from build123d import *
from build123d.topology import SkipClean

# Parameters (mm, degrees)
SKETCH2_R           = 18.921523051
SKETCH2_R_2         = 3.4
BOSS_EXTRUDE1_DEPTH = 10
FILLET1_R           = 3
SKETCH3_R           = 18.921523051
SKETCH3_R_2         = 3.4
BOSS_EXTRUDE2_DEPTH = 0.5
SKETCH4_R           = 18.921523051
BOSS_EXTRUDE3_DEPTH = 5
SKETCH8_R           = 18.921523051
BOSS_EXTRUDE4_DEPTH = 15
SKETCH10_R          = 4.25
CUT_EXTRUDE2_DEPTH  = 40
FILLET2_R           = 10
SKETCH11_R          = 3.4
CUT_EXTRUDE3_DEPTH  = 10.5


with BuildPart() as part:
    # Sketch2 → Boss-Extrude1 (new body)
    with BuildSketch(Plane.XY):
        Circle(SKETCH2_R)
        with Locations((0, 11.25277675)):
            Circle(SKETCH2_R_2, mode=Mode.SUBTRACT)
        with Locations((11.25277675, 0)):
            Circle(SKETCH2_R_2, mode=Mode.SUBTRACT)
        with Locations((0, -11.25277675)):
            Circle(SKETCH2_R_2, mode=Mode.SUBTRACT)
        with Locations((-11.25277675, 0)):
            Circle(SKETCH2_R_2, mode=Mode.SUBTRACT)
    extrude(amount=BOSS_EXTRUDE1_DEPTH)

    # Fillet1
    fillet1_edges = [part.edges().sort_by_distance(p)[0] for p in [
        (-18.921523051, 0, 0),
    ]]
    fillet(fillet1_edges, radius=FILLET1_R)

    # Sketch3 → Boss-Extrude2 (add)
    with BuildSketch(Plane.XY.offset(10)):
        Circle(SKETCH3_R)
        with Locations((0, 11.25277675)):
            Circle(SKETCH3_R_2, mode=Mode.SUBTRACT)
        with Locations((11.25277675, 0)):
            Circle(SKETCH3_R_2, mode=Mode.SUBTRACT)
        with Locations((-11.25277675, 0)):
            Circle(SKETCH3_R_2, mode=Mode.SUBTRACT)
        with Locations((0, -11.25277675)):
            Circle(SKETCH3_R_2, mode=Mode.SUBTRACT)
    extrude(amount=BOSS_EXTRUDE2_DEPTH)

    # Sketch4 → Boss-Extrude3 (add)
    with BuildSketch(Plane.XY.offset(10.5)):
        Circle(SKETCH4_R)
    extrude(amount=BOSS_EXTRUDE3_DEPTH)

    # Sketch8 → Boss-Extrude4 (add)
    with BuildSketch(Plane.XY.offset(15.5)):
        Circle(SKETCH8_R)
    extrude(amount=BOSS_EXTRUDE4_DEPTH)

    # Sketch9 → Revolve2 (revolve)
    with SkipClean():  # the faces are left unmerged after this step: merging them gives an invalid solid
        with BuildSketch(Plane.XY.offset(30.5)):
            with BuildLine():
                Line((0, -18.921523051), (0, 0))
                Line((0, 0), (0, 18.921523051))
                ThreePointArc((0, 18.921523051), (-18.921523051, 0), (0, -18.921523051))
            make_face()
            with BuildLine():
                Line((0, 18.921523051), (0, 0))
                Line((0, 0), (0, -18.921523051))
                ThreePointArc((0, -18.921523051), (13.37953726, -13.37953726), (18.921523051, 0))
                ThreePointArc((18.921523051, 0), (13.37953726, 13.37953726), (0, 18.921523051))
            make_face()
            with BuildLine():
                Line((0, 30), (0, 18.921523051))
                ThreePointArc((0, 18.921523051), (13.37953726, 13.37953726), (18.921523051, 0))
                ThreePointArc((18.921523051, 0), (13.37953726, -13.37953726), (0, -18.921523051))
                Line((0, -18.921523051), (0, -30))
                ThreePointArc((0, -30), (30, 0), (0, 30))
            make_face()
        revolve(axis=Axis((0, 0, 30.5), (0, 1, 0)))
    add(part.part.scale(1), mode=Mode.REPLACE)  # the faces are merged on a copy

    # Sketch10 → Cut-Extrude2 (cut)
    with BuildSketch(Plane(origin=(0, 0, 0), x_dir=(-1, 0, 0), z_dir=(0, 0, -1))):
        Circle(SKETCH10_R)
    extrude(amount=-CUT_EXTRUDE2_DEPTH, mode=Mode.SUBTRACT)

    # Fillet2
    fillet2_edges = [part.edges().sort_by_distance(p)[0] for p in [
        (-18.921523048, 0, 7.219622739),
    ]]
    fillet(fillet2_edges, radius=FILLET2_R)

    # Sketch11 → Cut-Extrude3 (cut)
    with SkipClean():  # the faces are left unmerged after this step: merging them gives an invalid solid
        with BuildSketch(Plane(origin=(0, 0, 0), x_dir=(-1, 0, 0), z_dir=(0, 0, -1))):
            with Locations((0, -11.25277675)):
                Circle(SKETCH11_R)
            with Locations((-11.25277675, 0)):
                Circle(SKETCH11_R)
            with Locations((0, 11.25277675)):
                Circle(SKETCH11_R)
            with Locations((11.25277675, 0)):
                Circle(SKETCH11_R)
        extrude(amount=-CUT_EXTRUDE3_DEPTH, mode=Mode.SUBTRACT)
    add(part.part.scale(1), mode=Mode.REPLACE)  # the faces are merged on a copy


solid = part.part
Could you check a few things on this model? Use its own coordinates, in mm. Coordinates: 2 decimals unless noted, no trailing zeros. Order: outer loops, then holes, each group sorted by start corner. A loop starts at its lowest first (then second) coordinate and runs counter-clockwise, first axis right, second up. Notation, with made-up numbers: (-30.75, 34) -> (21.25, 34) arc R12 cw to (21.25, 54) -> close; hole circle Ø10 at (-23.5, 32.25). An arc over 180 degrees is marked (long way). One line per question, with ' | ' between items.
Q1. Thinking about a two-plate mould opening in Y: for faces 1 (the face through (11, 0, 10.5)), 2 (the face through (-2.285, 3.584, 19.72)), 3 (the face through (3.3, -3.3, 0)), which applies, pulls with the +Y half, pulls with the -Y half, needs draft (parallel to the pull), parting line crosses it, or undercut?
Return value:
face 1: undercut | face 2: undercut | face 3: needs draft
Q2. Imagine slicing it at B-B on x = -24.5. Please give me the cut outline in (y, z), and give its area (3 significant figures).
Return value:
outline: circle Ø34.63 at (0, 30.5) | area: 942 mm²
Q3. Imagine slicing it at C-C on z = 43.5. Please give me the cut outline in (x, y).
Return value:
outline: circle Ø54.07 at (0, 0)
Q4. If I drill on L1, parallel to Y at x = 0, z = 4.75; L2, parallel to Y at x = 0, z = 7.25; L3, parallel to X at y = -14, z = 3, over which ranges is the centre line in solid material (lowest first)?
Return value:
L1: -19.1 to -14.65, -7.85 to -4.25, 4.25 to 7.85, 14.65 to 19.1 | L2: -19.93 to -14.65, -7.85 to -4.25, 4.25 to 7.85, 14.65 to 19.93 | L3: -12.73 to -2, 2 to 12.73
Q5. Imagine slicing it at A-A on z = 12.5. Please give me the cut outline in (x, y).
Return value:
outline: circle Ø48 at (0, 0); hole circle Ø8.5 at (0, 0)
Q6. I'm going to push flat-ended pins straight in: P1, Ø2, axis at x = -14, z = 7.5, coming from the -Y side; P2, Ø8, axis at x = 2, y = 6.5, coming from the -Z side; P3, Ø6, axis at x = 2, z = 27, coming from the +Y side; P4, Ø8, axis at x = -3, y = -23.5, coming from the -Z side. Where does each tip first touch, or does it pass through?
Return value:
P1: y = -15.56 | P2: z = 0 | P3: y = 29.98 | P4: z = 6.71
Q7. Imagine slicing it at D-D on z = 6. State how many separate pieces and enclosed holes the cut face has, and give its area (3 significant figures).
Return value:
separate pieces: 1 | enclosed holes: 5 | area: 983 mm²
